from build123d import *

# Parameters (mm, degrees)
F0_W     = 79
F0_H     = 84
F0_W_2   = 175
F0_H_2   = 35
F1_DEPTH = 5
F2_R     = 5
F3_R     = 5
F6_D     = 4.1
F8_D     = 49
F9_D     = 11


# Not quite as in the source:
# - a feature names something its author has since deleted; it is built from what else it names


with BuildPart() as f1:
    # F0 (on Top) → F1 (new body)
    with BuildSketch(Plane.XY):
        Polygon((-87.5, 50), (-117.5, 50), (-355, -15), (-355, -50), (-276, -50), (276, -50), (355, -50), (355, -15), (117.5, 50), (87.5, 50), align=None)
        with Locations((-315.5, -92)):
            Rectangle(F0_W, F0_H)
        with Locations((315.5, -92)):
            Rectangle(F0_W, F0_H)
        with Locations((0, 67.5)):
            Rectangle(F0_W_2, F0_H_2)
    extrude(amount=F1_DEPTH)

    # F2
    f2_edges = [f1.edges().sort_by_distance(p)[0] for p in [
        (-355, -134, 2.5),
        (-276, -134, 2.5),
        (276, -134, 2.5),
        (355, -134, 2.5),
        (355, -15, 2.5),
        (-355, -15, 2.5),
        (-276, -50, 2.5),
        (276, -50, 2.5),
        (-87.5, 50, 2.5),
        (-87.5, 85, 2.5),
        (87.5, 85, 2.5),
        (87.5, 50, 2.5),
    ]]
    fillet(f2_edges, radius=F2_R)

    # F3
    f3_edges = [f1.edges().sort_by_distance(p)[0] for p in [
        (117.5, 50, 2.5),
        (-117.5, 50, 2.5),
    ]]
    fillet(f3_edges, radius=F3_R)

    # F6 (through all)
    with Locations(Plane(origin=(0, 0, 0), x_dir=(1, 0, 0), z_dir=(0, 0, -1))):
        with Locations((-31, -17.5), (31, -17.5)):
            Hole(F6_D / 2)

    # F8 (through all)
    with Locations(Plane(origin=(0, 0, 0), x_dir=(1, 0, 0), z_dir=(0, 0, -1))):
        with Locations((-315.5, 97), (315.5, 97)):
            Hole(F8_D / 2)

    # F9 (through all)
    with Locations(Plane(origin=(0, 0, 0), x_dir=(1, 0, 0), z_dir=(0, 0, -1))):
        with Locations((-67.5, -68.5), (67.5, -68.5), (-26.5, -68.5), (26.5, -68.5), (-26.5, 33.5), (26.5, 33.5)):
            Hole(F9_D / 2)


solid = f1.part
Here's how the part is built. I have some questions about the finished solid (model axes, mm). Give positions to 0.01 mm unless a question says otherwise; leave off trailing zeros. Write each loop counter-clockwise with the first axis right and the second up, starting at its lowest first coordinate (ties: lowest second). Pieces come first, ordered by that corner, then holes. Notation, with made-up numbers: (-10, 54.25) -> (39, 54.25) arc R35 cw to (39, 89.25) -> close; hole circle Ø3 at (53, 31). An arc over 180 degrees is marked (long way). Use one line per item in the form item = value. Start each with the question number.
1. Imagine slicing it at D-D on y = 5.5. List the corners of the cut face in (x, z) for me.
2. Imagine slicing it at C-C on x = -40.5. List the corners of the cut face in (y, z) for me.
3. Will these pins go through, and if not, where does the flat tip stop? pin 1 Ø1.5 at (y, z) = (68, 2.5) entering from -X; pin 2 Ø1.5 at (y, z) = (66.5, 3) entering from +X; pin 3 Ø1 at (x, z) = (-11, 4) entering from -Y; pin 4 Ø14.5 at (x, y) = (67.5, 68.5) entering from +Z.
4. If I drill on L1, parallel to X at y = 68.5, z = 1.4; L2, parallel to Y at x = 26.5, z = 2.95; L3, parallel to Y at x = 67.5, z = 3.7, over which ranges is the centre line in solid material (lowest first)?
5. Imagine slicing it at A-A on y = -108. List the corners of the cut face in (x, z) for me.
6. Thinking about a two-plate mould opening in X: for faces 1 (the face through (-5, 1, 5)), 2 (the face through (-233.102, 18.362, 2.465)), 3 (the face through (-291.024, -98.077, 2.535)), which applies, +X half, -X half, draft (parallel to the pull), parting line (faces both ways), or undercut?
7. Imagine slicing it at B-B on z = 3.55. State how many separate pieces and enclosed holes the cut face has, plus the area to 3 significant figures.
Entries:
q1.outline = (-280.1, 0) -> (280.1, 0) -> (280.1, 5) -> (-280.1, 5) -> close
q2.outline = (-50, 0) -> (85, 0) -> (85, 5) -> (-50, 5) -> close
q3.pin_1 = -87.5
q3.pin_2 = 87.5
q3.pin_3 = -50
q3.pin_4 = 5
q4.L1 = -87.5 to -73, -62 to -32, -21 to 21, 32 to 62, 73 to 87.5
q4.L2 = -50 to -39, -28 to 63, 74 to 85
q4.L3 = -50 to 63, 74 to 85
q5.outline = (-355, 0) -> (-337.39, 0) -> (-337.39, 5) -> (-355, 5) -> close; (-293.61, 0) -> (-276, 0) -> (-276, 5) -> (-293.61, 5) -> close; (276, 0) -> (293.61, 0) -> (293.61, 5) -> (276, 5) -> close; (337.39, 0) -> (355, 0) -> (355, 5) -> (337.39, 5) -> close
q6.face_1 = draft
q6.face_2 = -X half
q6.face_3 = undercut
q7.separate_pieces = 1
q7.enclosed_holes = 10
q7.area = 70,600 mm²
